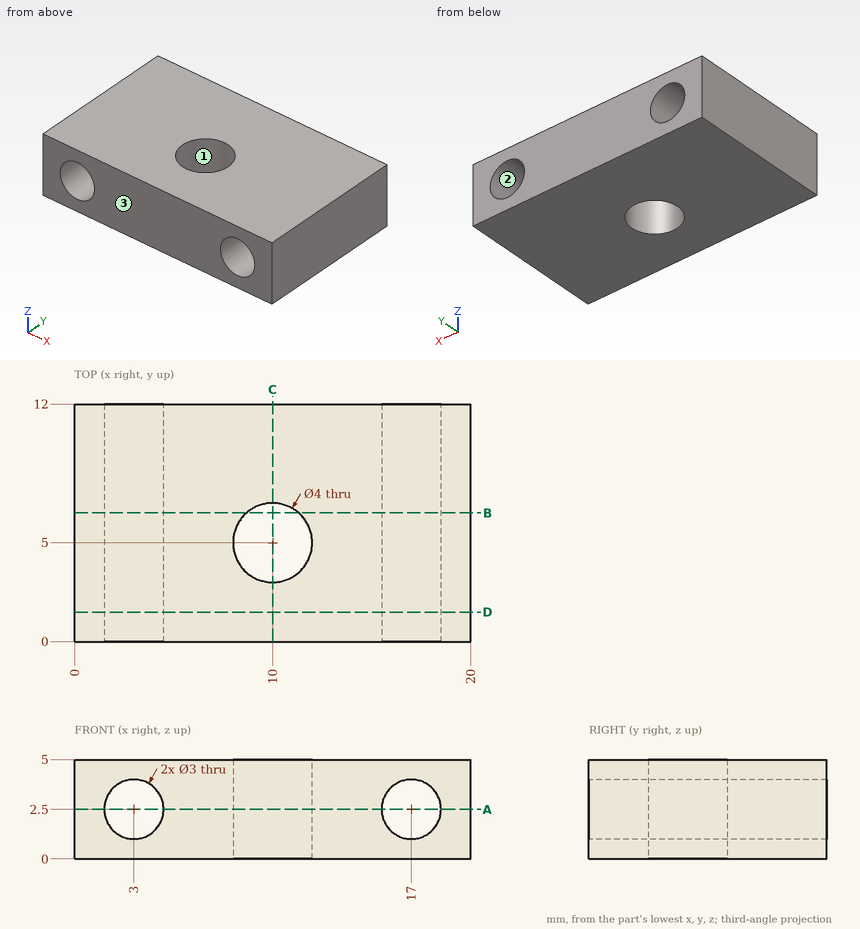
Here's the drawing with two shaded views (mm, measured from the low corner). I have some questions. Give positions to 0.01 mm unless a question says otherwise; leave off trailing zeros. Write each loop counter-clockwise with the first axis right and the second up, starting at its lowest first coordinate (ties: lowest second). Pieces come first, ordered by that corner, then holes. Notation, with made-up numbers: (88, 19) - (139, 19) arc R23 cw to (139, 52) - close; hole circle Ø5 at (-30, 57.5). An arc over 180 degrees is marked (long way). One line per item, written item: value. Start each with the question number.
Item 1: Imagine slicing it at B-B, the plane y = 6.5. List the corners of the cut face in (x, z) for me.
Item 2: I'm going to push a flat-ended pin straight in: pin 1 (2 mm diameter, centred on y = 8.5, z = 3, fed in from -X). Where does the tip first touch, or does it pass through?
Item 3: Imagine slicing it at D-D, the plane y = 1.5. List the corners of the cut face in (x, z) for me, and give its area (3 significant figures).
Item 4: Imagine slicing it at A-A, the plane z = 2.5. List the corners of the cut face in (x, y) for me, and give its area (3 significant figures).
Item 5: Please list where these lines run through material, in increasing order: line 1 (Z direction, x = 17, y = 7.75); line 2 (X direction, y = 0.5, z = 3.7); line 3 (X direction, y = 5.5, z = 1.65). Write a range as from..to.
Item 6: Imagine slicing it at C-C, the plane x = 10. List the corners of the cut face in (y, z) for me.
Item 7: If we mould it in two halves opening along Y, with no side actions, what happens to the marked faces 1, 2 and 3? For each: +Y half, -Y half, draft (parallel to the pull), parting line (faces both ways), or undercut.
Geometry says:
1. outline: (0, 0) - (8.68, 0) - (8.68, 5) - (0, 5) - close; (11.32, 0) - (20, 0) - (20, 5) - (11.32, 5) - close; hole circle Ø3 at (3, 2.5); hole circle Ø3 at (17, 2.5)
2. pin 1: x = 0
3. outline: (0, 0) - (20, 0) - (20, 5) - (0, 5) - close; hole circle Ø3 at (3, 2.5); hole circle Ø3 at (17, 2.5)
3. area: 85.9 mm^2
4. outline: (0, 0) - (1.5, 0) - (1.5, 12) - (0, 12) - close; (4.5, 0) - (15.5, 0) - (15.5, 12) - (4.5, 12) - close; (18.5, 0) - (20, 0) - (20, 12) - (18.5, 12) - close; hole circle Ø4 at (10, 5)
4. area: 155 mm^2
5. line 1: 0..1, 4..5
5. line 2: 0..2.1, 3.9..16.1, 17.9..20
5. line 3: 0..1.76, 4.24..8.06, 11.94..15.76, 18.24..20
6. outline: (0, 0) - (3, 0) - (3, 5) - (0, 5) - close; (7, 0) - (12, 0) - (12, 5) - (7, 5) - close
7. face 1: undercut
7. face 2: draft
7. face 3: -Y half
